Input: dimensioned drawing with shaded views. Units: mm. Origin: part minimum x, y, z. A direction names the side the tool comes from. Give positions to 0.01 mm unless a question says otherwise; leave off trailing zeros. Write each loop counter-clockwise with the first axis right and the second up, starting at its lowest first coordinate (ties: lowest second). Pieces come first, ordered by that corner, then holes. Notation, with made-up numbers: M 36.5,2.25 L 46.5,2.25 A21 cw 46.5,16.25 Z; hole C 44,-27.75 d8. An arc over 180 degrees is marked long. Answer as a JSON object with one key per item and string values.
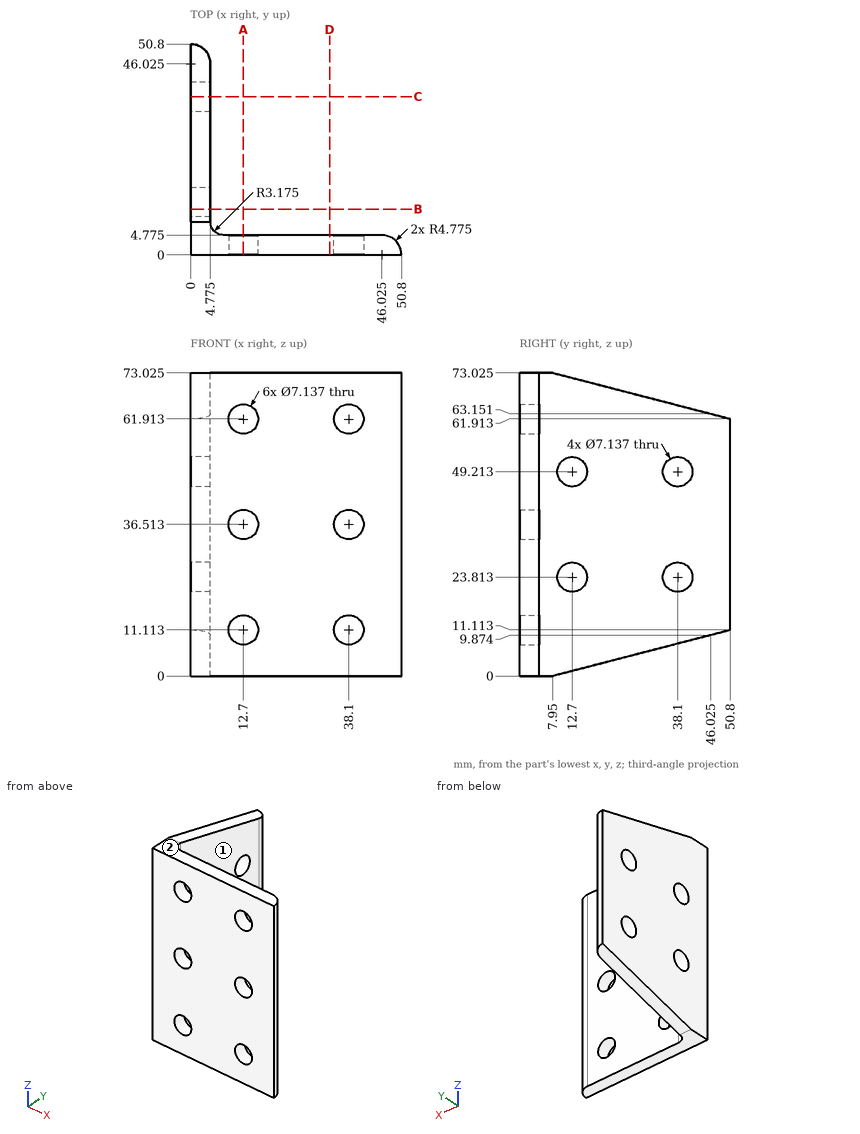
1) Cut plane C-C on y = 38.1. Return loops of the section in (x, z) (1 decimal).
Geometry check:
{"outline": "M 0,7.8 L 4.8,7.8 L 4.8,20.2 L 0,20.2 Z; M 0,27.4 L 4.8,27.4 L 4.8,45.6 L 0,45.6 Z; M 0,52.8 L 4.8,52.8 L 4.8,65.2 L 0,65.2 Z"}
2) Set-up query: the marked faces 1 and 2. Return all of +Z, -Z, +X, -X, +Y, -Y with unobstructed straight access to the full face (end or side cutting, diameter ignored); none if empty.
Geometry check:
{"face 1": "+Z, -Z, +X, +Y", "face 2": "+Z, +X, -X, +Y, -Y"}
3) Line query: line 1 (Z direction, x = 3.25, y = 12.7) (1 decimal); line 2 (Y direction, x = 34, z = 55.5) (1 decimal). Output: solid intervals per line, ascending. Write a range as from..to.
Geometry check:
{"line 1": "z = 1.2..20.2, 27.4..45.6, 52.8..71.8", "line 2": "y = 0..4.8"}
4) Contact query for flat-ended pins moving along their axis: P1, Ø5.5, axis at x = 38.1, z = 61.91, coming from the -Y side; P2, Ø12, axis at x = 8, y = 33.5, coming from the -Z side; P3, Ø1, axis at x = 45, z = 32.5, coming from the +Y side (1 decimal). Output: stop coordinate, or through.
Geometry check:
{"P1": "passes through", "P2": "stops at z = 5.31", "P3": "stops at y = 4.8"}
5) Cut plane B-B on y = 11. Give the number of separate pieces and of enclosed holes in the cut face, and give its area (3 significant figures).
Geometry check:
{"separate pieces": "3", "enclosed holes": "0", "area": "281 mm2"}
6) Cut plane D-D on x = 33.5. Return loops of the section in (y, z) (1 decimal).
Geometry check:
{"outline": "M 0,0 L 4.8,0 L 4.8,73 L 0,73 Z"}
7) Cut plane A-A on x = 12.7. Return loops of the section in (y, z) (1 decimal).
Geometry check:
{"outline": "M 0,0 L 4.8,0 L 4.8,7.5 L 0,7.5 Z; M 0,14.7 L 4.8,14.7 L 4.8,32.9 L 0,32.9 Z; M 0,40.1 L 4.8,40.1 L 4.8,58.3 L 0,58.3 Z; M 0,65.5 L 4.8,65.5 L 4.8,73 L 0,73 Z"}
